Source: CAD feature listing. Evaluate the final solid. Frame: model axes, mm. Face numbers are marked on the shaded views. A direction names the side the tool comes from. Give positions to 0.01 mm unless a question says otherwise; leave off trailing zeros. Write each loop counter-clockwise with the first axis right and the second up, starting at its lowest first coordinate (ties: lowest second). Pieces come first, ordered by that corner, then holes. Notation, with made-up numbers: (-0.75, 75) -> (30.25, 75) arc R20 ccw to (30.25, 99) -> close; hole circle Ø11 at (76, 88). An arc over 180 degrees is marked (long way). Use one line per item in the form item = value. Start each with the question number.
(1) Cut plane B-B, the plane x = 69. Output: boundary loops of the cut face in (y, z).
(2) Cut plane A-A, the plane y = 8.75. Output: boundary loops of the cut face in (x, z), and give its area (3 significant figures).
(3) First-contact query: P1, Ø12, axis at x = 65.5, z = -20, coming from the +Y side; P2, Ø1.5, axis at y = 25, z = 0, coming from the +X side; P3, Ø6, axis at x = 69.5, z = -39, coming from the +Y side. Flat tips, straight axial feed; report the tip coordinate or a pass-through.
(4) Cut plane C-C, the plane z = 18.5. Output: boundary loops of the cut face in (x, y).
(5) Material intervals for line 1 along Z through (x, y) = (61, 21.75); line 2 along X through (y, z) = (18.25, 3); line 3 along Z through (x, y) = (-23, 23.25), sorted ascending. Write a range as from..to.
(6) Cut plane D-D, the plane y = 16.5. Output: boundary loops of the cut face in (x, z).
(7) Set-up query: the marked faces 1 and 2. Return all of +Z, -Z, +X, -X, +Y, -Y with unobstructed straight access to the full face (end or side cutting, diameter ignored); none if empty.
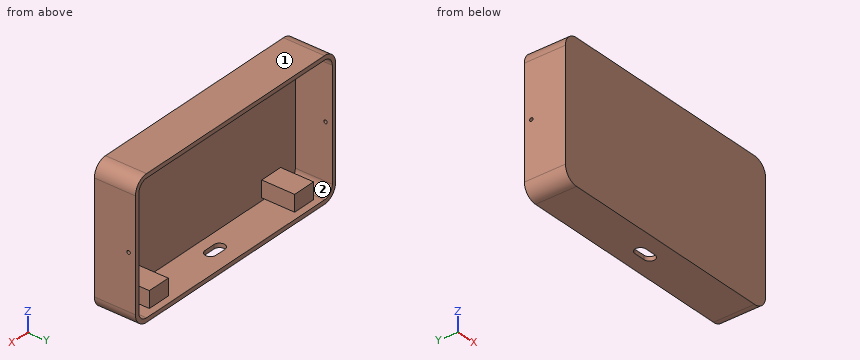
Autodesk Fusion 360 part; units mm, degrees
sketch "Walls" plane through (0, 0, 0) normal (0, 1, 0) x (1, 0, 0)
  line L0 (-80, 50) -> (80, 50)
  line L1 (90, 40) -> (90, -40)
  line L2 (80, -50) -> (-80, -50)
  line L3 (-90, -40) -> (-90, 40)
  line L4 (-90, 50) -> (90, -50) construction
  line L5 (90, 50) -> (-90, -50) construction
  arc A0 (-90, -40) -> (-80, -50) centre (-80, -40) ccw
  arc A1 (80, -50) -> (90, -40) centre (80, -40) ccw
  arc A2 (90, 40) -> (80, 50) centre (80, 40) ccw
  arc A3 (-80, 50) -> (-90, 40) centre (-80, 40) ccw
  arc A4 (87, 40) -> (80, 47) centre (80, 40) ccw
  line L6 (-80, 47) -> (80, 47)
  arc A5 (-80, 47) -> (-87, 40) centre (-80, 40) ccw
  line L7 (-87, -40) -> (-87, 40)
  arc A6 (-87, -40) -> (-80, -47) centre (-80, -40) ccw
  line L8 (80, -47) -> (-80, -47)
  arc A7 (80, -47) -> (87, -40) centre (80, -40) ccw
  line L9 (87, 40) -> (87, -40)
  dimension "d1" = 180
  dimension "d2" = 100
  dimension "d3" = 10
  dimension "d4" = 3
extrude "Floor Extrusion" add sketch "Walls" along normal blind 3 contours L0 L1 L2 L3 A0 A1 A2 A3 | A4 L6 A5 L7 A6 L8 A7 L9
extrude "Walls Extrusion" add sketch "Walls" along normal blind 30
sketch "Port" plane through (0, 0, -50) normal (0, 0, -1) x (-1, 0, 0)
  line L0 (-80, 0) -> (80, 0)
  line L1 (80, 0) -> (80, 30)
  line L2 (80, 30) -> (-80, 30)
  line L3 (-80, 30) -> (-80, 0)
  line L4 (4, 19) -> (-4, 19)
  arc A0 (-4, 19) -> (-4, 11) centre (-4, 15) ccw
  line L5 (-4, 11) -> (4, 11)
  arc A1 (4, 11) -> (4, 19) centre (4, 15) ccw
  line L6 (4, 15) -> (-4, 15) construction
  line L7 (80, 0) -> (-80, 0)
  dimension "d11" = 8
  dimension "d12" = 8
  dimension "d25" = 4
  dimension "d42" = 15
extrude "Port Extrusion" cut sketch "Port" against normal blind 3 contours L4 A0 L5 A1
sketch "Tab Holes" plane through (0, 0, 0) normal (1, 0, 0) x (0, 0, -1)
  circle A0 centre (0, 25) radius 1.25
  line L0 (-40, 30) -> (40, 30)
  dimension "d26" = 2.5
  dimension "d27" = 5
extrude "Tab Holes Extrusion" cut sketch "Tab Holes" along normal through all and the other way through all
sketch "Encoder Blocks" plane through (0, 3, 0) normal (0, 1, 0) x (-1, 0, 0)
  line L0 (87, -40) -> (87, 40)
  arc A0 (87, 40) -> (80, 47) centre (80, 40) ccw
  line L1 (80, 47) -> (-80, 47)
  arc A1 (-80, 47) -> (-87, 40) centre (-80, 40) ccw
  line L2 (-87, 40) -> (-87, -40)
  arc A2 (-87, -40) -> (-80, -47) centre (-80, -40) ccw
  line L3 (-80, -47) -> (80, -47)
  arc A3 (80, -47) -> (87, -40) centre (80, -40) ccw
  line L4 (73.8, -45) -> (56.8, -45)
  line L5 (56.8, -45) -> (56.8, -33)
  line L6 (56.8, -33) -> (73.8, -33)
  line L7 (73.8, -33) -> (73.8, -45)
  line L8 (73.8, -45) -> (56.8, -33) construction
  line L9 (56.8, -45) -> (73.8, -33) construction
  line L10 (80, -50) -> (-80, -50)
  line L11 (90, 40) -> (90, -40)
  line L12 (-56.8, -45) -> (-73.8, -33) construction
  line L13 (-56.8, -33) -> (-56.8, -45)
  line L14 (-56.8, -45) -> (-73.8, -45)
  line L15 (-73.8, -45) -> (-56.8, -33) construction
  line L16 (-73.8, -33) -> (-56.8, -33)
  line L17 (-73.8, -45) -> (-73.8, -33)
  line L18 (80, -47) -> (-80, -47)
  line L19 (-90, -40) -> (-90, 40)
  point P0 (65.3, -39)
  point P1 (-65.3, -39)
  dimension "d29" = 17
  dimension "d30" = 12
  dimension "d31" = 5
  dimension "d32" = 16.2
  dimension "d35" = 17
  dimension "d36" = 12
  dimension "d38" = 5
  dimension "d39" = 16.2
extrude "Left Encoder Block Extrusion" add sketch "Encoder Blocks" along normal blind 24 contours L4 L5 L6 L7
extrude "Right Encoder Block Extrusion" add sketch "Encoder Blocks" along normal blind 24 contours L13 L14 L16 L17
equation "d25 = ( 8 / 2 ) * 1 mm"
equation "d27 = ( 10 / 2 ) * 1 mm"
equation "d33 = 30 mm - 3 mm - 3 mm"
equation "d40 = 30 mm - 3 mm - 3 mm"
equation "d42 = ( 30 / 2 ) * 1 mm"
Geometry says:
q1.outline = (0, -50) -> (30, -50) -> (30, -47) -> (3, -47) -> (3, -45) -> (27, -45) -> (27, -33) -> (3, -33) -> (3, 47) -> (30, 47) -> (30, 50) -> (0, 50) -> close
q2.outline = (-90, -40) arc R10 ccw to (-80, -50) -> (80, -50) arc R10 ccw to (90, -40) -> (90, 40) arc R10 ccw to (80, 50) -> (-80, 50) arc R10 ccw to (-90, 40) -> close; (-73.8, -45) -> (-56.8, -45) -> (-56.8, -33) -> (-73.8, -33) -> close; (56.8, -45) -> (73.8, -45) -> (73.8, -33) -> (56.8, -33) -> close; hole (-87, -40) arc R7 ccw to (-80, -47) -> (80, -47) arc R7 ccw to (87, -40) -> (87, 40) arc R7 ccw to (80, 47) -> (-80, 47) arc R7 ccw to (-87, 40) -> close
q2.area = 2,010 mm^2
q3.P1 = 3
q3.P2 = through
q3.P3 = 27
q4.outline = (-90, 0) -> (90, 0) -> (90, 30) -> (87, 30) -> (87, 3) -> (-87, 3) -> (-87, 30) -> (-90, 30) -> close
q5.line_1 = -50..-47, -45..-33, 47..50
q5.line_2 = -90..-87, 87..90
q5.line_3 = -50..-47, 47..50
q6.outline = (-90, -40) arc R10 ccw to (-80, -50) -> (-7.71, -50) -> (-7.71, -47) -> (-80, -47) arc R7 cw to (-87, -40) -> (-87, 40) arc R7 cw to (-80, 47) -> (80, 47) arc R7 cw to (87, 40) -> (87, -40) arc R7 cw to (80, -47) -> (7.71, -47) -> (7.71, -50) -> (80, -50) arc R10 ccw to (90, -40) -> (90, 40) arc R10 ccw to (80, 50) -> (-80, 50) arc R10 ccw to (-90, 40) -> close; (-73.8, -45) -> (-56.8, -45) -> (-56.8, -33) -> (-73.8, -33) -> close; (56.8, -45) -> (73.8, -45) -> (73.8, -33) -> (56.8, -33) -> close
q7.face_1 = +Z, +X, -X, +Y, -Y
q7.face_2 = +Y
